```python
from build123d import *

# Parameters (mm, degrees)
F0_W     = 203.2
F0_H     = 203.2
F1_DEPTH = 254
F3_W     = 25.4
F3_H     = 203.2
F3_W_2   = 203.2
F4_DEPTH = 25.4
F5_D     = 76.2
F5_DEPTH = 127
F5_TIP   = 22.892789585
F6_W     = 101.6
F6_H     = 12.7
F7_DEPTH = 38.1


with BuildPart() as f1:
    # F0 (on Top) → F1 (new body)
    with BuildSketch(Plane.XY):
        with Locations((-101.6, 101.6)):
            Rectangle(F0_W, F0_H)
    extrude(amount=F1_DEPTH)

    # F3 (on face) → F4 (join)
    with BuildSketch(Plane.XY.offset(254)):
        with Locations((-215.9, 101.6)):
            Rectangle(F3_W, F3_H)
        with Locations((12.7, 101.6)):
            Rectangle(F3_W, F3_H)
        with Locations((-101.6, 101.6)):
            Rectangle(F3_W_2, F3_H)
    extrude(amount=F4_DEPTH)

    # F5
    with Locations(Plane.XZ):
        with Locations((-101.6, 108.5994392633)):
            Hole(F5_D / 2, depth=F5_DEPTH)
            with Locations((0, 0, -(F5_DEPTH + F5_TIP / 2))):  # 118° drill point
                Cone(0, F5_D / 2, F5_TIP, mode=Mode.SUBTRACT)

    # F6 (on face) → F7 (join)
    with BuildSketch(Plane.XZ):
        with Locations((-101.4467881441, 54.7498768032)):
            Rectangle(F6_W, F6_H)
    extrude(amount=F7_DEPTH)


solid = f1.part
```
Geometry: final body of the model. Coordinates: model frame, mm. A direction names the side the tool comes from. Give positions to 0.01 mm unless a question says otherwise; leave off trailing zeros. Write each loop counter-clockwise with the first axis right and the second up, starting at its lowest first coordinate (ties: lowest second). Pieces come first, ordered by that corner, then holes.
1. Section query A-A, the plane y = 47.5. Return loops of the section in (x, z).
2. Section query B-B, the plane x = -11.5. Return loops of the section in (y, z).
3. Draft query along Z for faces 1 (the conical face through (-98.043, 145.917, 114.179)), 2 (the flat face through (-228.6, 100, 267)), 3 (the flat face through (-103, 103, 279.4)). Return one class per face: released by +Z, released by -Z, zero draft, split by the parting line, or undercut.
4. Line query: probe 1 along Z at (x, y) = (-101.6, 88.5); probe 2 along X at (y, z) = (90.5, 244.5); probe 3 along Y at (x, z) = (-81.5, 172). Output: solid intervals per line, ascending.
5. Reachability of faces 4 (the flat face through (-203.2, 100, 125)), 5 (the flat face through (-102, -19, 61.1)), 6 (the cylindrical face through (-73.52, 64.39, 134.35)) from +Z, -Z, +X, -X, +Y, -Y: full face, straight path, thin tool, end or side. Return the list, or none.
6. Section query C-C, the plane z = 259.5. Return loops of the section in (x, y), then the cut area to 3 significant figures.
7. Pin query (flat end, axial travel): P1, Ø10, axis at y = -16.5, z = 51.5, coming from the -X side; P2, Ø14, axis at y = -14.5, z = 52.5, coming from the +X side; P3, Ø7.5, axis at x = 8, y = 89, coming from the -Z side. Return the tip coordinate at first contact, or that it passes through.
Computed:
1. outline: (-228.6, 254) - (-203.2, 254) - (-203.2, 0) - (0, 0) - (0, 254) - (25.4, 254) - (25.4, 279.4) - (-228.6, 279.4) - close; hole circle Ø76.2 at (-101.6, 108.6)
2. outline: (0, 0) - (203.2, 0) - (203.2, 279.4) - (0, 279.4) - close
3. face 1: undercut
3. face 2: zero draft
3. face 3: released by +Z
4. probe 1: z = 0 to 70.5, 146.7 to 279.4
4. probe 2: x = -203.2 to 0
4. probe 3: y = 0 to 203.2
5. face 4: -Z, -X, +Y, -Y
5. face 5: +Z, +X, -X, -Y
5. face 6: -Y
6. outline: (-228.6, 0) - (25.4, 0) - (25.4, 203.2) - (-228.6, 203.2) - close
6. area: 51,600 mm2
7. P1: stops at x = -152.25
7. P2: stops at x = -50.65
7. P3: stops at z = 254
